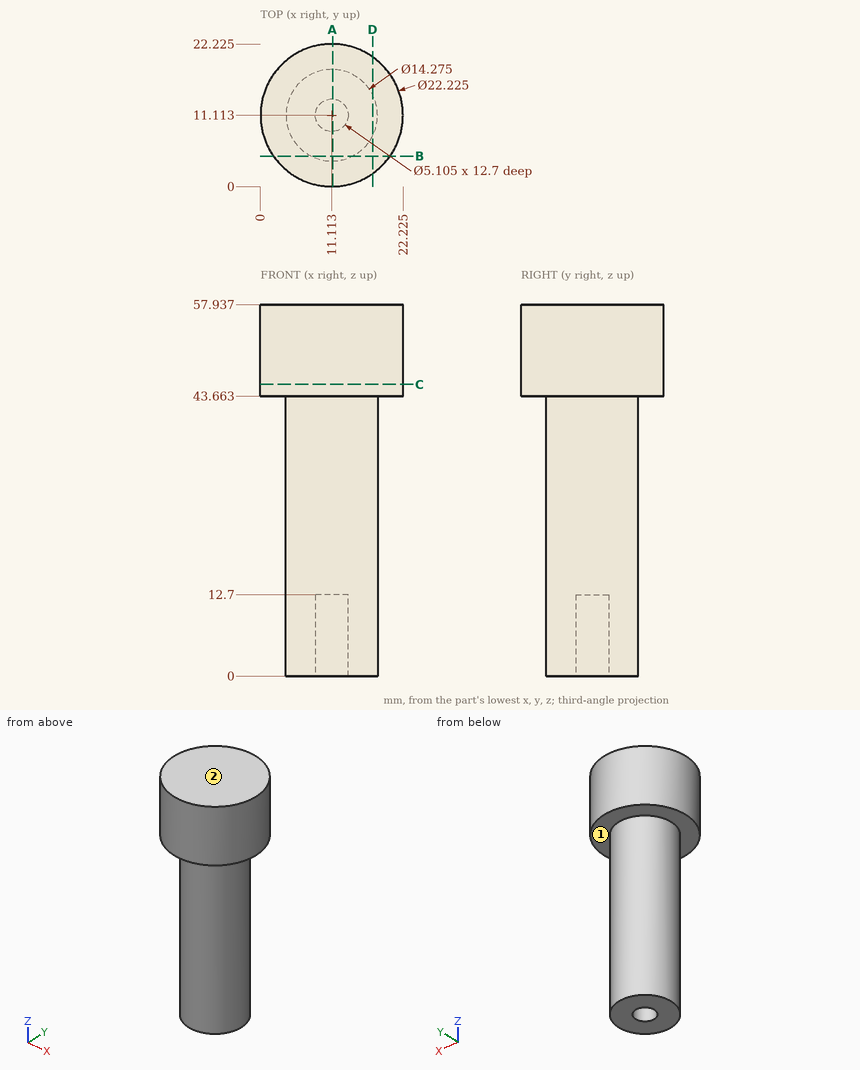
Geometry: see drawing. Coordinates: mm, zero at the bounding-box minimum. A direction names the side the tool comes from. Give positions to 0.01 mm unless a question says otherwise; leave off trailing zeros. Loops run counter-clockwise (first coordinate to the right, second up) from the corner with the lowest first, then second, coordinate; pieces in that order, holes last. Notation, with made-up numbers: (-14, -33.75) - (-2, -33.75) arc R21 cw to (-2, 5.25) - close; hole circle Ø9 at (7.25, 65.25). An arc over 180 degrees is marked (long way). Use CSV: the item, a comma, the result in double quotes.
1) Cut plane C-C (z = 45.5). Output: boundary loops of the cut face in (x, y) (1 decimal), and give its area (3 significant figures).
Worked out:
outline,"circle Ø22.2 at (11.1, 11.1)"
area,"388 mm^2"
2) Line query: line 1 (Z direction, x = 3.25, y = 5.75); line 2 (X direction, y = 9.5, z = 14.5) (1 decimal); line 3 (Y direction, x = 10, z = 17). Output: solid intervals per line, ascending.
Worked out:
line 1,"z = 43.66 to 57.94"
line 2,"x = 4.2 to 18.1"
line 3,"y = 4.06 to 18.16"
3) Cut plane B-B (y = 4.75). Output: boundary loops of the cut face in (x, z).
Worked out:
outline,"(2, 43.66) - (7.88, 43.66) - (7.88, 0) - (14.35, 0) - (14.35, 43.66) - (20.22, 43.66) - (20.22, 57.94) - (2, 57.94) - close"
4) Cut plane A-A (x = 11.25). Output: boundary loops of the cut face in (y, z) (1 decimal).
Worked out:
outline,"(0, 43.7) - (4, 43.7) - (4, 0) - (8.6, 0) - (8.6, 12.7) - (13.7, 12.7) - (13.7, 0) - (18.2, 0) - (18.2, 43.7) - (22.2, 43.7) - (22.2, 57.9) - (0, 57.9) - close"
5) Set-up query: the marked faces 1 and 2. Return all of +Z, -Z, +X, -X, +Y, -Y with unobstructed straight access to the full face (end or side cutting, diameter ignored); none if empty.
Worked out:
face 1,"-Z"
face 2,"+Z, +X, -X, +Y, -Y"
6) Pin query (flat end, axial travel): P1, Ø1.5, axis at y = 19, z = 49, coming from the -X side (1 decimal); P2, Ø6, axis at y = 6, z = 50.5, coming from the -X side; P3, Ø2.5, axis at x = 11.5, y = 10.5, coming from the -Z side. Return the tip coordinate at first contact, or that it passes through.
Worked out:
P1,"stops at x = 2.6"
P2,"stops at x = 0.2"
P3,"stops at z = 12.7"
7) Cut plane D-D (x = 17.5). Output: boundary loops of the cut face in (y, z) (1 decimal), and give its area (3 significant figures).
Worked out:
outline,"(2, 43.7) - (7.9, 43.7) - (7.9, 0) - (14.3, 0) - (14.3, 43.7) - (20.2, 43.7) - (20.2, 57.9) - (2, 57.9) - close"
area,"538 mm^2"
